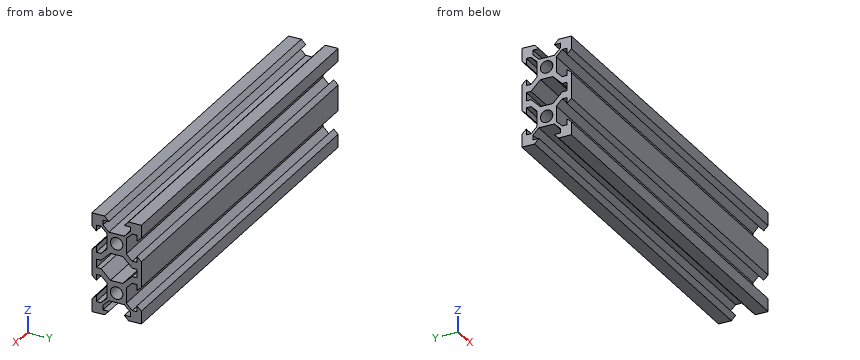
Autodesk Inventor part; units mm, degrees
ref_plane "YZ Plane" through (0, 0, 0) normal (1, 0, 0) x (0, 1, 0)
ref_plane "XZ Plane" through (0, 0, 0) normal (0, 1, 0) x (-1, 0, 0)
ref_plane "XY Plane" through (0, 0, 0) normal (0, 0, 1) x (1, 0, 0)
sketch "Sketch1" plane through (0, 0, 0) normal (1, 0, 0) x (0, 1, 0)
  line L0 (10, 20) -> (-10, 20)
  line L1 (-10, 20) -> (-10, -20)
  line L2 (-10, -20) -> (10, -20)
  line L3 (10, -20) -> (10, 20)
  line L4 (10, 20) -> (-10, -20) construction
  line L5 (-10, 20) -> (10, -20) construction
  line L6 (0, -20) -> (0, -10) construction
  circle A0 centre (0, -10) radius 2.5
  line L7 (10, 0) -> (0, 0) construction
  circle A1 centre (0, 10) radius 2.5
  line L8 (0, 20) -> (0, 18.2) construction
  line L9 (0, 18.2) -> (3.125, 18.2)
  line L10 (0, 18.2) -> (0, 13.9)
  line L11 (0, 20) -> (4.8, 20)
  line L12 (4.8, 20) -> (3.125, 18.2)
  line L13 (0, 18.2) -> (5.5, 18.2)
  line L14 (0, 13.9) -> (3.125, 13.9)
  line L15 (5.5, 18.2) -> (5.5, 16.275)
  line L16 (3.125, 13.9) -> (5.5, 16.275)
  line L17 (3.125, 13.9) -> (8.7353, 13.9) construction
  line L18 (0, 18.2) -> (-3.125, 18.2)
  line L19 (0, 20) -> (-4.8, 20)
  line L20 (-4.8, 20) -> (-3.125, 18.2)
  line L21 (0, 18.2) -> (-5.5, 18.2)
  line L22 (0, 13.9) -> (-3.125, 13.9)
  line L23 (-5.5, 18.2) -> (-5.5, 16.275)
  line L24 (-3.125, 13.9) -> (-5.5, 16.275)
  line L25 (10, 10) -> (8.2, 10) construction
  line L26 (8.2, 10) -> (8.2, 6.875)
  line L27 (8.2, 10) -> (3.9, 10)
  line L28 (10, 10) -> (10, 5.2)
  line L29 (10, 5.2) -> (8.2, 6.875)
  line L30 (8.2, 10) -> (8.2, 4.5)
  line L31 (3.9, 10) -> (3.9, 6.875)
  line L32 (8.2, 4.5) -> (6.275, 4.5)
  line L33 (3.9, 6.875) -> (6.275, 4.5)
  line L34 (3.9, 13.125) -> (6.275, 15.5)
  line L35 (8.2, 10) -> (8.2, 15.5)
  line L36 (8.2, 15.5) -> (6.275, 15.5)
  line L37 (8.2, 10) -> (8.2, 13.125)
  line L38 (10, 10) -> (10, 14.8)
  line L39 (10, 14.8) -> (8.2, 13.125)
  line L40 (3.9, 10) -> (3.9, 13.125)
  line L41 (0, 10) -> (10, 10) construction
  line L42 (-3.9, 10) -> (-3.9, 13.125)
  line L43 (-3.9, 13.125) -> (-6.275, 15.5)
  line L44 (-8.2, 10) -> (-8.2, 15.5)
  line L45 (-8.2, 15.5) -> (-6.275, 15.5)
  line L46 (-10, 14.8) -> (-8.2, 13.125)
  line L47 (-3.9, 10) -> (-3.9, 6.875)
  line L48 (-3.9, 6.875) -> (-6.275, 4.5)
  line L49 (-8.2, 4.5) -> (-6.275, 4.5)
  line L50 (-8.2, 10) -> (-8.2, 4.5)
  line L51 (-10, 5.2) -> (-8.2, 6.875)
  line L52 (0, -20) -> (0, -18.2) construction
  line L53 (0, -18.2) -> (3.125, -18.2)
  line L54 (0, -18.2) -> (0, -13.9)
  line L55 (0, -20) -> (4.8, -20)
  line L56 (4.8, -20) -> (3.125, -18.2)
  line L57 (0, -18.2) -> (5.5, -18.2)
  line L58 (0, -13.9) -> (3.125, -13.9)
  line L59 (5.5, -18.2) -> (5.5, -16.275)
  line L60 (3.125, -13.9) -> (5.5, -16.275)
  line L61 (3.125, -13.9) -> (8.7353, -13.9) construction
  line L62 (-3.125, -13.9) -> (-5.5, -16.275)
  line L63 (0, -18.2) -> (-5.5, -18.2)
  line L64 (-5.5, -18.2) -> (-5.5, -16.275)
  line L65 (0, -18.2) -> (-3.125, -18.2)
  line L66 (0, -20) -> (-4.8, -20)
  line L67 (-4.8, -20) -> (-3.125, -18.2)
  line L68 (0, -13.9) -> (-3.125, -13.9)
  line L69 (8.2, -10) -> (8.2, -13.125)
  line L70 (3.9, -10) -> (3.9, -13.125)
  line L71 (3.9, -13.125) -> (6.275, -15.5)
  line L72 (10, -10) -> (10, -14.8)
  line L73 (8.2, -10) -> (8.2, -15.5)
  line L74 (8.2, -15.5) -> (6.275, -15.5)
  line L75 (10, -14.8) -> (8.2, -13.125)
  line L76 (3.9, -10) -> (3.9, -6.875)
  line L77 (3.9, -6.875) -> (6.275, -4.5)
  line L78 (8.2, -4.5) -> (6.275, -4.5)
  line L79 (8.2, -10) -> (3.9, -10)
  line L80 (8.2, -10) -> (8.2, -6.875)
  line L81 (8.2, -10) -> (8.2, -4.5)
  line L82 (10, -5.2) -> (8.2, -6.875)
  line L83 (10, -10) -> (10, -5.2)
  line L84 (10, -10) -> (8.2, -10) construction
  line L85 (-10, -14.8) -> (-8.2, -13.125)
  line L86 (-8.2, -10) -> (-8.2, -15.5)
  line L87 (-8.2, -15.5) -> (-6.275, -15.5)
  line L88 (-3.9, -13.125) -> (-6.275, -15.5)
  line L89 (-3.9, -10) -> (-3.9, -13.125)
  line L90 (-3.9, -10) -> (-3.9, -6.875)
  line L91 (-3.9, -6.875) -> (-6.275, -4.5)
  line L92 (-8.2, -4.5) -> (-6.275, -4.5)
  line L93 (-8.2, -10) -> (-8.2, -4.5)
  line L94 (-10, -5.2) -> (-8.2, -6.875)
  line L95 (-8.2, -4.5) -> (-8.2, 0) construction
  line L96 (-8.2, 0) -> (-8.2, 1.7)
  line L97 (-8.2, 1.7) -> (-6.275, 1.7)
  line L98 (-6.275, 1.7) -> (-2.5, 5.475)
  line L99 (-3.9, 6.875) -> (-1.2394, 4.2144) construction
  line L100 (-2.5, 5.475) -> (2.5, 5.475)
  line L101 (3.9, 6.875) -> (1.5625, 4.5375) construction
  line L102 (-6.275, 1.7) -> (13.7612, 1.7) construction
  line L103 (-6.275, 1.7) -> (13.7612, 1.7) construction
  line L104 (2.5, 5.475) -> (6.275, 1.7)
  line L105 (6.275, 1.7) -> (8.2, 1.7)
  line L106 (8.2, 1.7) -> (8.2, 0)
  line L107 (-8.2, 0) -> (-8.2, -1.7)
  line L108 (-8.2, -1.7) -> (-6.275, -1.7)
  line L109 (-6.275, -1.7) -> (-2.5, -5.475)
  line L110 (-2.5, -5.475) -> (2.5, -5.475)
  line L111 (2.5, -5.475) -> (6.275, -1.7)
  line L112 (6.275, -1.7) -> (8.2, -1.7)
  line L113 (8.2, -1.7) -> (8.2, 0)
  point P0 (10, -10)
  dimension "d0" = 20
  dimension "d1" = 40
  dimension "d2" = 10
  dimension "d3" = 5
  dimension "d4" = 10
  dimension "d5" = 1.8
  dimension "d6" = 3.125
  dimension "d7" = 4.3
  dimension "d9" = 4.8
  dimension "d11" = 5.5
  dimension "d12" = 3.125
  dimension "d13" = 45
  dimension "d14" = 1.8
  dimension "d15" = 3.125
  dimension "d16" = 4.3
  dimension "d17" = 4.8
  dimension "d18" = 5.5
  dimension "d19" = 3.125
  dimension "d20" = 1.7
  dimension "d21" = 0
extrude "Extrusion1" add sketch "Sketch1" along normal blind 150 contours L3 L39 L35 L36 L34 L40 L31 L33 L32 L30 L29 L82 L81 L78 L77 L76 L70 L71 L74 L73 L75 L2 L56 L57 L59 L60 L58 L68 L62 L64 L63 L67 L1 L85 L86 L87 L88 L89 L90 L91 L92 L93 L94 L51 L50 L49 L48 L47 L42 L43 L45 L44 L46 L0 L20 L21 L23 L24 L22 L14 L16 L15 L13 L12
properties part number "VSLOT"
Geometry check sheet. Reference: the model listing, model coordinates, mm. Round coordinates to 2 decimals unless told otherwise and drop trailing zeros. Loops run counter-clockwise (first coordinate to the right, second up) from the corner with the lowest first, then second, coordinate; pieces in that order, holes last.
Item 1: Thickness scan on line 1 (Z direction, x = 55.5, y = 0) (3 decimals); line 2 (Z direction, x = 74.5, y = -7.75); line 3 (Y direction, x = 55, z = -18). Record the ranges inside material, lowest first.
Item 2: Gauge pin test, flat ends, axial feed: pin 1 (5 mm diameter, centred on x = 98, z = -11, fed in from -Y); pin 2 (1.2 mm diameter, centred on x = 78.5, z = -14, fed in from +Y); pin 3 (3 mm diameter, centred on x = 78, z = 11, fed in from -Y). Record the tip position at first contact, or that the pin passes through.
Item 3: Cross-section at A-A on y = 0. Record the boundary of the cut face in (x, z) (3 decimals).
Item 4: Cross-section at C-C on x = 129. Count the separate pieces of the cut face and the enclosed holes in it, then the cut area to 3 significant figures.
Item 5: Cross-section at B-B on z = 10. Record the boundary of the cut face in (x, y).
Answer sheet:
1. line 1: z = -13.9 to -12.5, -7.5 to -5.475, 5.475 to 7.5, 12.5 to 13.9
1. line 2: z = -20 to -15.5, -4.5 to -1.7, 1.7 to 4.5, 15.5 to 20
1. line 3: y = -10 to -5.5, 5.5 to 10
2. pin 1: stops at y = -8.6
2. pin 2: stops at y = 9.79
2. pin 3: stops at y = -3.9
3. outline: (0, -13.9) - (150, -13.9) - (150, -12.5) - (0, -12.5) - close; (0, -7.5) - (150, -7.5) - (150, -5.475) - (0, -5.475) - close; (0, 5.475) - (150, 5.475) - (150, 7.5) - (0, 7.5) - close; (0, 12.5) - (150, 12.5) - (150, 13.9) - (0, 13.9) - close
4. separate pieces: 1
4. enclosed holes: 3
4. area: 303 mm2
5. outline: (0, -3.9) - (150, -3.9) - (150, -2.5) - (0, -2.5) - close; (0, 2.5) - (150, 2.5) - (150, 3.9) - (0, 3.9) - close
